from build123d import *

# Parameters (mm, degrees)
F0_R     = 10
F1_DEPTH = 30


with BuildPart() as f1:
    # F0 (on Front) → F1 (new body)
    with BuildSketch(Plane.XZ):
        with BuildLine():
            ThreePointArc((-38.37657, -29.162996), (-36.912104, -32.698529), (-33.37657, -34.162996))
            Line((-33.37657, -34.162996), (31.62343, -34.162996))
            Line((31.62343, -34.162996), (31.62343, -19.162996))
            Line((31.62343, -19.162996), (41.720804, -8.070519))
            Line((41.720804, -8.070519), (35.292928, -0.410074))
            Line((35.292928, -0.410074), (23.802262, -10.051889))
            Line((23.802262, -10.051889), (17.374386, -2.391444))
            Line((17.374386, -2.391444), (29.541973, 7.818374))
            Line((29.541973, 7.818374), (23.114097, 15.478819))
            Line((23.114097, 15.478819), (11.62343, 5.837004))
            Line((11.62343, 5.837004), (1.62343, 5.837004))
            Line((1.62343, 5.837004), (1.62343, -4.162996))
            Line((1.62343, -4.162996), (-3.37657, -4.162996))
            Line((-3.37657, -4.162996), (-3.37657, 5.837004))
            Line((-3.37657, 5.837004), (-18.37657, 5.837004))
            ThreePointArc((-18.37657, 5.837004), (-21.912104, 4.372538), (-23.37657, 0.837004))
            Line((-23.37657, 0.837004), (-23.37657, -14.162996))
            Line((-23.37657, -14.162996), (-33.37657, -14.162996))
            ThreePointArc((-33.37657, -14.162996), (-36.912104, -15.627462), (-38.37657, -19.162996))
            Line((-38.37657, -19.162996), (-38.37657, -29.162996))
        make_face()
        with Locations((-2.191618, -19.162996)):
            Circle(F0_R, mode=Mode.SUBTRACT)
    extrude(amount=F1_DEPTH)


solid = f1.part
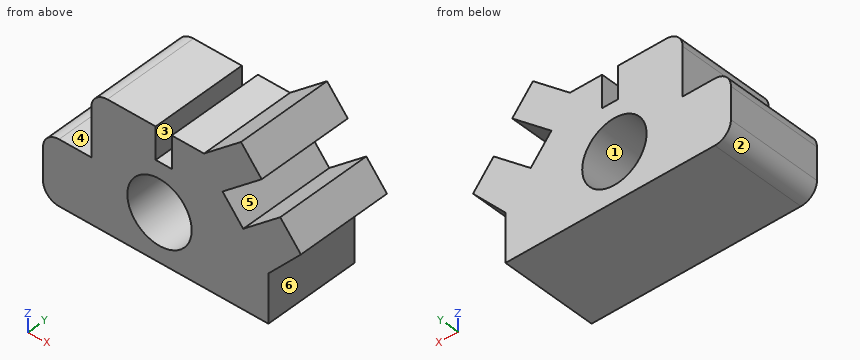
Can you work these out from the model? Positions are in its coordinate system, mm. Face numbers are marked on the shaded views. A direction names the side the tool comes from. Coordinates: 2 decimals unless noted, no trailing zeros. Write each loop counter-clockwise with the first axis right and the second up, starting at its lowest first coordinate (ties: lowest second). Pieces come first, ordered by that corner, then holes. Notation, with made-up numbers: (-25.75, 37.5) -> (15.25, 37.5) arc R11 ccw to (15.25, 57.5) -> close; hole circle Ø2 at (80.5, 26). An arc over 180 degrees is marked (long way). Write each question's results on one line, items separated by ' | '. Start each with the question number.
Item 1: If we section it at B-B, the plane x = 21: Write out the boundary of the cut face in (y, z).
Item 2: If we section it at A-A, the plane y = -16.25: Write out the boundary of the cut face in (x, z).
Item 3: If we section it at D-D, the plane x = 9: Write out the boundary of the cut face in (y, z).
Item 4: On a 3-axis mill with a long thin cutter (end or side, diameter ignored), from which of +Z, -Z, +X, -X, +Y, -Y can I reach the whole of each face in a straight line? I mean the marked faces 4, 5 and 6. Say none if no direction works.
Item 5: If we section it at C-C, the plane z = -25: Write out the boundary of the cut face in (x, y).
Item 6: Thinking about a two-plate mould opening in Z: for the marked faces 1, 2 and 3, which applies, released by +Z, released by -Z, zero draft, split by the parting line, or undercut?
Item 7: Please list where these lines run through material, in increasing order: probe 1 along X at (y, z) = (-28.5, -3); probe 2 along Z at (x, y) = (9, -22.5); probe 3 along X at (y, z) = (-13.25, -28).
Item 8: I'm going to push flat-ended pins straight in: P1, Ø12, axis at y = -18, z = -26, coming from the +X side; P2, Ø4.5, axis at x = -14, y = -11.5, coming from the +Z side; P3, Ø12, axis at y = -3.5, z = 6.5, coming from the +X side; P4, Ø12, axis at x = -2.19, z = -19.16, coming from the +Y side. Where does each tip first touch, or does it pass through?
Answer block:
1) outline: (-30, -34.16) -> (0, -34.16) -> (0, -6.71) -> (-30, -6.71) -> close; (-30, 0.65) -> (0, 0.65) -> (0, 13.7) -> (-30, 13.7) -> close
2) outline: (-38.38, -29.16) arc R5 ccw to (-33.38, -34.16) -> (31.62, -34.16) -> (31.62, -19.16) -> (41.72, -8.07) -> (35.29, -0.41) -> (23.8, -10.05) -> (17.37, -2.39) -> (29.54, 7.82) -> (23.11, 15.48) -> (11.62, 5.84) -> (1.62, 5.84) -> (1.62, -4.16) -> (-3.38, -4.16) -> (-3.38, 5.84) -> (-18.38, 5.84) arc R5 ccw to (-23.38, 0.84) -> (-23.38, -14.16) -> (-33.38, -14.16) arc R5 ccw to (-38.38, -19.16) -> close; hole circle Ø20 at (-2.19, -19.16)
3) outline: (-30, -34.16) -> (0, -34.16) -> (0, 5.84) -> (-30, 5.84) -> close
4) face 4: +Z, -X, +Y, -Y | face 5: +Y, -Y | face 6: -Z, +X, +Y, -Y
5) outline: (-38.38, -30) -> (-10.31, -30) -> (-10.31, 0) -> (-38.38, 0) -> close; (5.93, -30) -> (31.62, -30) -> (31.62, 0) -> (5.93, 0) -> close
6) face 1: undercut | face 2: released by -Z | face 3: zero draft
7) probe 1: -23.38 to -3.38, 1.62 to 17.89, 32.21 to 37.47 | probe 2: -34.16 to 5.84 | probe 3: -38.38 to -6.87, 2.49 to 31.62
8) P1: x = 31.62 | P2: z = 5.84 | P3: x = 29.54 | P4: through
